Check sheet for the modelled part. Datum: model origin and axes. Units: mm. Face numbers are marked on the shaded views. A direction names the side the tool comes from. Round coordinates to 2 decimals unless told otherwise and drop trailing zeros. Order: outer loops, then holes, each group sorted by start corner. A loop starts at its lowest first (then second) coordinate and runs counter-clockwise, first axis right, second up.
Q1. Set-up check for the marked faces 4, 5, 6, 7 and 8: record each of +Z, -Z, +X, -X, +Y, -Y from which the full face is reachable in a straight line by a thin tool's end or side.
Q2. Scan lines: probe 1 along Z at (x, y) = (70, -47.5); probe 2 along Y at (x, z) = (-1.5, 32); probe 3 along Z at (x, y) = (99, -4) (3 decimals). Record each from-to range of solid material in increasing order.
Q3. Cross-section at A-A on z = 1.5. Record the cut outline in (x, y) (3 decimals).
Q4. Cross-section at C-C on x = 98.5. Record the cut outline in (y, z) (3 decimals).
Q5. Mould release check, pull along X, two halves, no side actions. Record for the marked faces 1, 2 and 3: +X half, -X half, draft (parallel to the pull), parting line (faces both ways), or undercut.
Q6. Depth check by flat-ended pin: P1, Ø8, axis at x = 55, y = -9.5, coming from the -Z side; P2, Ø1, axis at y = 6.5, z = 30, coming from the +X side; P3, Ø4, axis at y = -45, z = 19, coming from the -X side (3 decimals). Enter the tip coordinate at first touch or a pass-through.
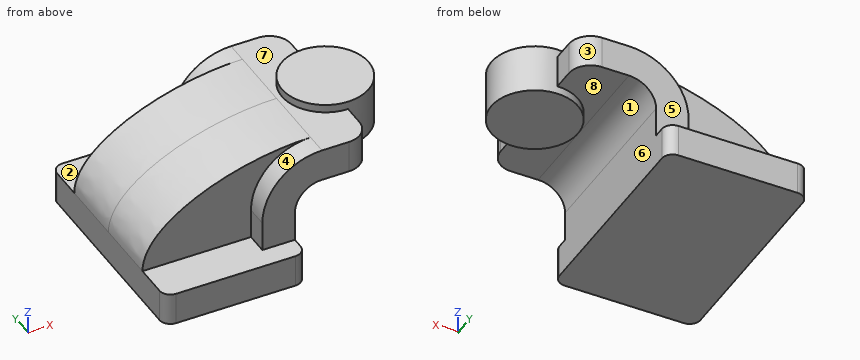
from build123d import *

# Parameters (mm, degrees)
F1_DEPTH = 63.5
F0_W     = 25.4
F0_H     = 19.05
F2_DEPTH = 50.8
F3_DEPTH = 38.1
F5_R     = 6.35
F6_R     = 12.7


with BuildPart() as f1:
    # F0 (on Front) → F1 (new body, symmetric)
    with BuildSketch(Plane.XZ):
        Polygon((22.225, 9.525), (-41.275, 9.525), (-41.275, -9.525), (41.275, -9.525), (41.275, 9.525), align=None)
    extrude(amount=F1_DEPTH, both=True)

    # F0 (on Front) → F2 (join, symmetric)
    with BuildSketch(Plane.XZ):
        with BuildLine():
            Line((22.225, 27.0002), (22.225, 9.525))
            Line((22.225, 9.525), (41.275, 9.525))
            Line((41.275, 9.525), (41.275, 27.0002))
            ThreePointArc((41.275, 27.0002), (45.9246798487, 38.2255201513), (57.15, 42.8752))
            Line((57.15, 42.8752), (60.325, 42.8752))
            Line((60.325, 42.8752), (60.325, 61.9252))
            Line((60.325, 61.9252), (57.15, 61.9252))
            ThreePointArc((57.15, 61.9252), (32.4542956671, 51.6959043329), (22.225, 27.0002))
        make_face()
        with Locations((73.025, 52.4002)):
            Rectangle(F0_W, F0_H)
    extrude(amount=F2_DEPTH, both=True)

    # F0 (on Front) → F3 (join, symmetric)
    with BuildSketch(Plane.XZ):
        with BuildLine():
            add(Edge.make_bspline(
                [(-41.275, 9.525), (-41.275, 38.7971624732), (11.6867609322, 61.9252), (57.15, 61.9252)],
                knots=[0, 0, 0, 0, 111.5045361635, 111.5045361635, 111.5045361635, 111.5045361635], degree=3))
            Line((-41.275, 9.525), (22.225, 9.525))
            Line((22.225, 9.525), (22.225, 27.0002))
            ThreePointArc((22.225, 27.0002), (32.4542956671, 51.6959043329), (57.15, 61.9252))
        make_face()
    extrude(amount=F3_DEPTH, both=True)

    # F0 (on Front) → F4 (revolve)
    with BuildSketch(Plane.XZ):
        Polygon((85.725, 66.675), (85.725, 61.9252), (85.725, 42.8752), (85.725, 38.1), (111.125, 38.1), (111.125, 66.675), align=None)
    revolve(axis=Axis((85.725, 0, 52.3875), (0, 0, 1)))

    # F5
    f5_edges = [f1.edges().sort_by_distance(p)[0] for p in [
        (41.275, -63.5, 0),
        (41.275, 63.5, 0),
        (-41.275, 63.5, 0),
        (-41.275, -63.5, 0),
    ]]
    fillet(f5_edges, radius=F5_R)

    # F6
    f6_edges = [f1.edges().sort_by_distance(p)[0] for p in [
        (85.725, -50.8, 52.4002),
        (85.725, 50.8, 52.4002),
    ]]
    fillet(f6_edges, radius=F6_R)


solid = f1.part
Results found:
1. face 4: +Z, -X, -Y
1. face 5: +Z, +X, -X, +Y
1. face 6: -Z, +X, +Y, -Y
1. face 7: +Z, -X
1. face 8: -Z
2. probe 1: z = 42.88 to 61.93
2. probe 2: y = -38.1 to 38.1
2. probe 3: z = 38.1 to 66.675
3. outline: (-41.275, -57.15) arc R6.35 ccw to (-34.925, -63.5) - (34.925, -63.5) arc R6.35 ccw to (41.275, -57.15) - (41.275, 57.15) arc R6.35 ccw to (34.925, 63.5) - (-34.925, 63.5) arc R6.35 ccw to (-41.275, 57.15) - close
4. outline: (-21.954, 38.1) - (21.954, 38.1) - (21.954, 66.675) - (-21.954, 66.675) - close
5. face 1: undercut
5. face 2: draft
5. face 3: +X half
6. P1: stops at z = 41.64
6. P2: stops at x = 41.67
6. P3: stops at x = 22.225
